from build123d import *

# Parameters (mm, degrees)
SKETCH2_R           = 3.175
BOSS_EXTRUDE1_DEPTH = 43.815
SKETCH5_R           = 1.27
CUT_EXTRUDE1_DEPTH  = 5.08
SKETCH6_R           = 1.27
CUT_EXTRUDE2_DEPTH  = 58.452587844
SKETCH7_W           = 28.702
SKETCH7_H           = 55.88
CUT_EXTRUDE3_DEPTH  = 5.08
SKETCH8_W           = 1.27
SKETCH8_H           = 5.08
CUT_EXTRUDE4_DEPTH  = 57.547097627


with BuildPart() as part:
    # Sketch2 → Boss-Extrude1 (new, symmetric)
    with BuildSketch(Plane(origin=(0, 0, 0), x_dir=(1, 0, 0), z_dir=(0, 1, 0))):
        with BuildLine():
            Line((-28.575, 6.35), (28.575, 6.35))
            ThreePointArc((28.575, 6.35), (34.925, 0), (28.575, -6.35))
            Line((28.575, -6.35), (-28.575, -6.35))
            ThreePointArc((-28.575, -6.35), (-34.925, 0), (-28.575, 6.35))
        make_face()
        with Locations(Location((28.575, 0, 0), (0, 0, 270))):
            Circle(SKETCH2_R, mode=Mode.SUBTRACT)
        with Locations(Location((-28.575, 0, 0), (0, 0, 270))):
            Circle(SKETCH2_R, mode=Mode.SUBTRACT)
    extrude(amount=BOSS_EXTRUDE1_DEPTH, both=True)

    # Sketch5 → Cut-Extrude1 (cut)
    with BuildSketch(Plane(origin=(0, 0, -6.35), x_dir=(-1, 0, 0), z_dir=(0, 0, -1))):
        with Locations((22.86, 36.83)):
            Circle(SKETCH5_R)
        with Locations((22.86, 20.32)):
            Circle(SKETCH5_R)
        with Locations((-22.86, 36.83)):
            Circle(SKETCH5_R)
        with Locations((-22.86, 20.32)):
            Circle(SKETCH5_R)
    extrude(amount=-CUT_EXTRUDE1_DEPTH, mode=Mode.SUBTRACT)

    # Sketch6 → Cut-Extrude2 (cut, through all)
    with BuildSketch(Plane.XY.offset(6.35)):
        with Locations(Location((22.86, 36.83, 0), (0, 0, 180))):
            Circle(SKETCH6_R)
        with Locations(Location((22.86, 20.32, 0), (0, 0, 180))):
            Circle(SKETCH6_R)
        with Locations(Location((-22.86, 36.83, 0), (0, 0, 180))):
            Circle(SKETCH6_R)
        with Locations(Location((-22.86, 20.32, 0), (0, 0, 180))):
            Circle(SKETCH6_R)
    extrude(amount=-CUT_EXTRUDE2_DEPTH, mode=Mode.SUBTRACT)

    # Sketch7 → Cut-Extrude3 (cut)
    with BuildSketch(Plane.XY.offset(6.35)):
        with Locations((0, -12.7)):
            Rectangle(SKETCH7_W, SKETCH7_H)
    cut_extrude3 = extrude(amount=-CUT_EXTRUDE3_DEPTH, mode=Mode.SUBTRACT)

    # Mirror1: Cut-Extrude3 across plane
    add(cut_extrude3.mirror(Plane.XY), mode=Mode.SUBTRACT)

    # Sketch8 → Cut-Extrude4 (cut, through all)
    with BuildSketch(Plane.XY.offset(1.27)):
        with Locations((13.716, -33.02)):
            Rectangle(SKETCH8_W, SKETCH8_H)
        with Locations((13.716, -2.54)):
            Rectangle(SKETCH8_W, SKETCH8_H)
    cut_extrude4 = extrude(amount=-CUT_EXTRUDE4_DEPTH, mode=Mode.SUBTRACT)

    # Mirror2: Cut-Extrude4 across plane
    add(cut_extrude4.mirror(Plane(origin=(0, 0, 0), x_dir=(0, 0, 1), z_dir=(1, 0, 0))), mode=Mode.SUBTRACT)


solid = part.part
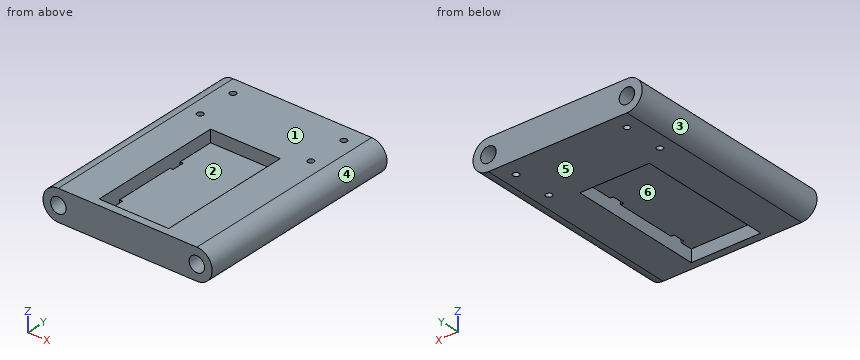
Could you check a few things on this model? Use its own coordinates, in mm. Face numbers are marked on the shaded views. A direction names the side the tool comes from. Give positions to 0.01 mm unless a question says otherwise; leave off trailing zeros. Write each loop counter-clockwise with the first axis right and the second up, starting at its lowest first coordinate (ties: lowest second). Pieces come first, ordered by that corner, then holes. Notation, with made-up numbers: (28.25, 8.25) -> (34.25, 8.25) arc R11 ccw to (34.25, 13.25) -> close; hole circle Ø9 at (-15, 39.25). An arc over 180 degrees is marked (long way). Write each question's results on one line, items separated by ' | '. Start each with the question number.
Q1. We'd pull the mould along X, two halves only. Please class the marked faces 1, 2, 3 and 4: +X half, -X half, draft (parallel to the pull), parting line (faces both ways), or undercut.
Q2. Which directions (+Z, -Z, +X, -X, +Y, -Y) give clear straight access to the entire face, cutting with the end or side of a thin tool? Please do the marked faces 5 and 6.
Q3. Suppose I cut it at C-C, the plane x = 22.86. List the corners of the cut face in (y, z) for me (3 decimals).
Q4. Suppose I cut it at A-A, the plane z = 0. State how many separate pieces and enclosed holes the cut face has, and give its area (3 significant figures).
Q5. I need wall thicknesses on probe 1 along Y at (x, z) = (-22.86, -1) (3 decimals); probe 2 along X at (y, z) = (-9, 0) (3 decimals); probe 3 along X at (y, z) = (20.32, 1). Which ranges of each line are inside material? Lowest first, please.
Q6. I'm going to push flat-ended pins straight in: pin 1 Ø8 at (x, y) = (8.5, -29) entering from +Z; pin 2 Ø8 at (x, y) = (6.5, -32.5) entering from -Z. Where does each tip first touch, or does it pass through?
Q7. Suppose I cut it at B-B, the plane y = 36.83. List the corners of the cut face in (x, z) for me (3 decimals), and give its area (3 significant figures).
Q8. Suppose I cut it at D-D, the plane y = 9.5. List the corners of the cut face in (x, z) for me (3 decimals).
Outcome:
1) face 1: draft | face 2: undercut | face 3: -X half | face 4: +X half
2) face 5: -Z, +X, -X, +Y, -Y | face 6: -Z
3) outline: (-43.815, -6.35) -> (19.05, -6.35) -> (19.05, 6.35) -> (-43.815, 6.35) -> close; (21.59, -6.35) -> (35.56, -6.35) -> (35.56, 6.35) -> (21.59, 6.35) -> close; (38.1, -6.35) -> (43.815, -6.35) -> (43.815, 6.35) -> (38.1, 6.35) -> close
4) separate pieces: 3 | enclosed holes: 8 | area: 4,960 mm2
5) probe 1: -43.815 to 19.05, 21.59 to 35.56, 38.1 to 43.815 | probe 2: -34.925 to -31.75, -25.4 to 25.4, 31.75 to 34.925 | probe 3: -34.85 to -31.59, -25.56 to -24.13, -21.59 to 21.59, 24.13 to 25.56, 31.59 to 34.85
6) pin 1: z = 1.27 | pin 2: z = -1.27
7) outline: (-28.575, -6.35) -> (-24.13, -6.35) -> (-24.13, 6.35) -> (-28.575, 6.35) arc R6.35 ccw to start; (-21.59, -6.35) -> (21.59, -6.35) -> (21.59, 6.35) -> (-21.59, 6.35) -> close; (24.13, -6.35) -> (28.575, -6.35) arc R6.35 ccw to (28.575, 6.35) -> (24.13, 6.35) -> close; hole circle Ø6.35 at (-28.575, 0); hole circle Ø6.35 at (28.575, 0) | area: 725 mm2
8) outline: (-28.575, -6.35) -> (-14.351, -6.35) -> (-14.351, -1.27) -> (14.351, -1.27) -> (14.351, -6.35) -> (28.575, -6.35) arc R6.35 ccw to (28.575, 6.35) -> (14.351, 6.35) -> (14.351, 1.27) -> (-14.351, 1.27) -> (-14.351, 6.35) -> (-28.575, 6.35) arc R6.35 ccw to start; hole circle Ø6.35 at (-28.575, 0); hole circle Ø6.35 at (28.575, 0)
